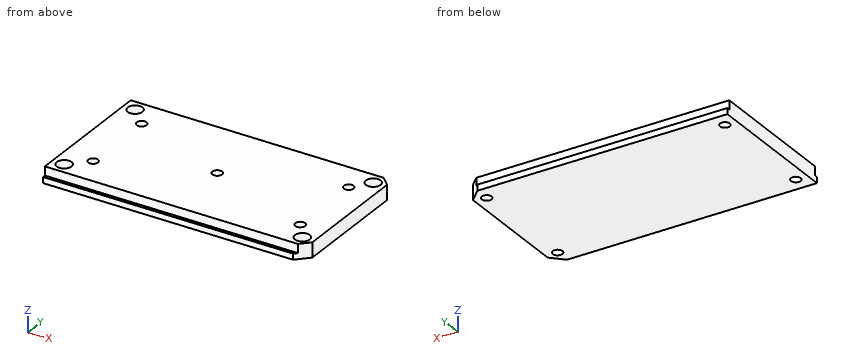
```python
from build123d import *

# Parameters (mm, degrees)
F0_W      = 88.5
F0_H      = 46
F1_DEPTH  = 5
F2_R      = 2.5
F6_DEPTH  = 3
F3_R      = 2.5
F7_DEPTH  = 3
F4_R      = 2.5
F8_DEPTH  = 3
F5_R      = 2.5
F9_DEPTH  = 3
F12_R     = 1.65
F14_DEPTH = 3
F13_R     = 1.65
F15_DEPTH = 3
F11_R     = 1.65
F16_DEPTH = 3
F10_R     = 1.65
F17_DEPTH = 3
F18_R     = 1.65
F19_DEPTH = 4
F20_R     = 1.65
F21_R     = 1.65
F24_DEPTH = 4
F22_R     = 1.65
F23_R     = 1.65
F25_DEPTH = 4
F26_W     = 88.5
F26_H     = 2
F27_DEPTH = 1
F28_W     = 88.5
F28_H     = 2
F29_DEPTH = 1
F30_SIZE  = 3
F32_DEPTH = 3
F33_SIZE  = 3
F35_DEPTH = 3


with BuildPart() as f1:
    # F0 (on Top) → F1 (new body)
    with BuildSketch(Plane.XY):
        with Locations((44.25, 23)):
            Rectangle(F0_W, F0_H)
    extrude(amount=F1_DEPTH)

    # F2 (on face) → F6 (cut)
    with BuildSketch(Plane.XY.offset(5)):
        with Locations((4, 42)):
            Circle(F2_R)
    extrude(amount=-F6_DEPTH, mode=Mode.SUBTRACT)

    # F3 (on face) → F7 (cut)
    with BuildSketch(Plane.XY.offset(5)):
        with Locations((4, 4)):
            Circle(F3_R)
    extrude(amount=-F7_DEPTH, mode=Mode.SUBTRACT)

    # F4 (on face) → F8 (cut)
    with BuildSketch(Plane.XY.offset(5)):
        with Locations((84.5, 42)):
            Circle(F4_R)
    extrude(amount=-F8_DEPTH, mode=Mode.SUBTRACT)

    # F5 (on face) → F9 (cut)
    with BuildSketch(Plane.XY.offset(5)):
        with Locations((84.5, 4)):
            Circle(F5_R)
    extrude(amount=-F9_DEPTH, mode=Mode.SUBTRACT)

    # F12 (on face) → F14 (cut)
    with BuildSketch(Plane.XY.offset(2)):
        with Locations((84.5, 42)):
            Circle(F12_R)
    extrude(amount=-F14_DEPTH, mode=Mode.SUBTRACT)

    # F13 (on face) → F15 (cut)
    with BuildSketch(Plane.XY.offset(2)):
        with Locations((84.5, 4)):
            Circle(F13_R)
    extrude(amount=-F15_DEPTH, mode=Mode.SUBTRACT)

    # F11 (on face) → F16 (cut)
    with BuildSketch(Plane.XY.offset(2)):
        with Locations((4, 4)):
            Circle(F11_R)
    extrude(amount=-F16_DEPTH, mode=Mode.SUBTRACT)

    # F10 (on face) → F17 (cut)
    with BuildSketch(Plane.XY.offset(2)):
        with Locations((4, 42)):
            Circle(F10_R)
    extrude(amount=-F17_DEPTH, mode=Mode.SUBTRACT)

    # F18 (on face) → F19 (cut)
    with BuildSketch(Plane.XY.offset(5)):
        with Locations((43.75, 23)):
            Circle(F18_R)
    extrude(amount=-F19_DEPTH, mode=Mode.SUBTRACT)

    # F20 (on face) + F21 (on face) → F24 (cut)
    with BuildSketch(Plane.XY.offset(5)):
        with Locations((10, 36)):
            Circle(F20_R)
    with BuildSketch(Plane.XY.offset(5)):
        with Locations((10, 10)):
            Circle(F21_R)
    extrude(amount=-F24_DEPTH, mode=Mode.SUBTRACT)

    # F22 (on face) + F23 (on face) → F25 (cut)
    with BuildSketch(Plane.XY.offset(5)):
        with Locations((80, 36)):
            Circle(F22_R)
    with BuildSketch(Plane.XY.offset(5)):
        with Locations((80, 10)):
            Circle(F23_R)
    extrude(amount=-F25_DEPTH, mode=Mode.SUBTRACT)

    # F26 (on face) → F27 (join)
    with BuildSketch(Plane(origin=(0, 46, 0), x_dir=(-1, 0, 0), z_dir=(0, 1, 0))):
        with Locations((-44.25, 1)):
            Rectangle(F26_W, F26_H)
    extrude(amount=F27_DEPTH)

    # F28 (on face) → F29 (join)
    with BuildSketch(Plane.XZ):
        with Locations((44.25, 1)):
            Rectangle(F28_W, F28_H)
    extrude(amount=F29_DEPTH)

    # F30
    f30_edges = [f1.edges().sort_by_distance(p)[0] for p in [
        (88.5, 0, 3.5),
    ]]
    chamfer(f30_edges, length=F30_SIZE)

    # F31 (on face) → F32 (cut)
    with BuildSketch(Plane.XY.offset(2)):
        Polygon((88.5, 0), (88.5, 3), (85.5, 0), (84.5, -1), (88.5, -1), align=None)
    extrude(amount=-F32_DEPTH, mode=Mode.SUBTRACT)

    # F33
    f33_edges = [f1.edges().sort_by_distance(p)[0] for p in [
        (88.5, 46, 3.5),
    ]]
    chamfer(f33_edges, length=F33_SIZE)

    # F34 (on face) → F35 (cut)
    with BuildSketch(Plane.XY.offset(2)):
        Polygon((85.5, 46), (88.5, 43), (88.5, 46), (88.5, 47), (84.5, 47), align=None)
    extrude(amount=-F35_DEPTH, mode=Mode.SUBTRACT)


solid = f1.part
```
Input: part model. Units: mm. Frame: model coordinates. Coordinates: 2 decimals unless noted, no trailing zeros. Write each loop counter-clockwise with the first axis right and the second up, starting at its lowest first coordinate (ties: lowest second). Pieces come first, ordered by that corner, then holes.
1) Section D-D on y = 36. Output: boundary loops of the cut face in (x, z).
2) Pin query (flat end, axial travel): pin 1 Ø2.5 at (x, y) = (10, 10) entering from +Z; pin 2 Ø1.5 at (x, y) = (84.5, 5) entering from +Z; pin 3 Ø1 at (x, z) = (29.5, 3) entering from -Y. Return the tip coordinate at first contact, or that it passes through.
3) Section B-B on x = 80. Output: boundary loops of the cut face in (y, z), and give its area (3 significant figures).
4) Section A-A on y = 4. Output: boundary loops of the cut face in (x, z).
5) Material intervals for line 1 along Y through (x, z) = (4, 3.35); line 2 along Y through (x, z) = (80, 3.6); line 3 along X through (y, z) = (11.5, 1.4), sorted ascending.
6) Section C-C on x = 4. Output: boundary loops of the cut face in (y, z).
Check result:
1. outline: (0, 0) - (88.5, 0) - (88.5, 5) - (81.65, 5) - (81.65, 1) - (78.35, 1) - (78.35, 5) - (11.65, 5) - (11.65, 1) - (8.35, 1) - (8.35, 5) - (0, 5) - close
2. pin 1: stops at z = 1
2. pin 2: stops at z = 2
2. pin 3: stops at y = 0
3. outline: (-1, 0) - (47, 0) - (47, 2) - (46, 2) - (46, 5) - (37.65, 5) - (37.65, 1) - (34.35, 1) - (34.35, 5) - (11.65, 5) - (11.65, 1) - (8.35, 1) - (8.35, 5) - (0, 5) - (0, 2) - (-1, 2) - close
3. area: 208 mm2
4. outline: (0, 0) - (2.35, 0) - (2.35, 2) - (1.5, 2) - (1.5, 5) - (0, 5) - close; (5.65, 0) - (82.85, 0) - (82.85, 2) - (82, 2) - (82, 5) - (6.5, 5) - (6.5, 2) - (5.65, 2) - close; (86.15, 0) - (88.5, 0) - (88.5, 5) - (87, 5) - (87, 2) - (86.15, 2) - close
5. line 1: y = 0 to 1.5, 6.5 to 39.5, 44.5 to 46
5. line 2: y = 0 to 8.35, 11.65 to 34.35, 37.65 to 46
5. line 3: x = 0 to 9.31, 10.69 to 79.31, 80.69 to 88.5
6. outline: (-1, 0) - (2.35, 0) - (2.35, 2) - (1.5, 2) - (1.5, 5) - (0, 5) - (0, 2) - (-1, 2) - close; (5.65, 0) - (40.35, 0) - (40.35, 2) - (39.5, 2) - (39.5, 5) - (6.5, 5) - (6.5, 2) - (5.65, 2) - close; (43.65, 0) - (47, 0) - (47, 2) - (46, 2) - (46, 5) - (44.5, 5) - (44.5, 2) - (43.65, 2) - close
